```python
from build123d import *

# Parameters (mm, degrees)
SKETCH1_W                      = 40
SKETCH1_H                      = 31
SKETCH1_R                      = 8.75
BOSS_EXTRUDE1_DEPTH            = 19
SHELL1_T                       = -2
SKETCH2_R                      = 10.75
SKETCH2_R_2                    = 8.75
CUT_EXTRUDE1_DEPTH             = 14.5
SKETCH3_W                      = 2
SKETCH3_H                      = 5
BOSS_EXTRUDE2_DEPTH            = 17
SKETCH8_W                      = 7
SKETCH8_H                      = 7
BOSS_EXTRUDE3_DEPTH            = 3
CBORE_FOR_M3_SHCS1_D           = 3.4
CBORE_FOR_M3_SHCS1_CBORE_D     = 6.5
CBORE_FOR_M3_SHCS1_CBORE_DEPTH = 3
CUT_EXTRUDE3_REACH             = 46.125


with BuildPart() as part:
    # Sketch1 → Boss-Extrude1 (new body)
    with BuildSketch(Plane.XY):
        with Locations((-5, 0)):
            Rectangle(SKETCH1_W, SKETCH1_H)
        Circle(SKETCH1_R, mode=Mode.SUBTRACT)
    extrude(amount=-BOSS_EXTRUDE1_DEPTH)

    # Shell1
    shell1_openings = [part.faces().sort_by_distance(p)[0] for p in [
        (-5, -14.993936763, 0),
    ]]
    offset(amount=SHELL1_T, openings=shell1_openings, kind=Kind.INTERSECTION)

    # Sketch2 → Cut-Extrude1 (cut)
    with BuildSketch(Plane.XY):
        with Locations(Location((0, 0, 0), (0, 0, 180))):
            Circle(SKETCH2_R)
        Circle(SKETCH2_R_2, mode=Mode.SUBTRACT)
    extrude(amount=-CUT_EXTRUDE1_DEPTH, mode=Mode.SUBTRACT)

    # Sketch3 → Boss-Extrude2 (add)
    with BuildSketch(Plane.XY.offset(-17)):
        with Locations((-19, 11)):
            Rectangle(SKETCH3_W, SKETCH3_H)
    extrude(amount=BOSS_EXTRUDE2_DEPTH)

    # Sketch8 → Boss-Extrude3 (add)
    with BuildSketch(Plane.XY.offset(-17)):
        with Locations((-14.5, 10)):
            Rectangle(SKETCH8_W, SKETCH8_H)
    extrude(amount=BOSS_EXTRUDE3_DEPTH)

    # CBORE for M3 SHCS1 (through all)
    with Locations(Plane(origin=(0, 0, -19), x_dir=(-1, 0, 0), z_dir=(0, 0, -1))):
        with Locations((15, 10.5)):
            CounterBoreHole(CBORE_FOR_M3_SHCS1_D / 2, CBORE_FOR_M3_SHCS1_CBORE_D / 2, CBORE_FOR_M3_SHCS1_CBORE_DEPTH)

    # Sketch9 → Cut-Extrude3 (cut, up to next)
    with BuildSketch(Plane.XZ.offset(15.5), mode=Mode.PRIVATE) as cut_extrude3_sk1:
        Polygon((-12, 0), (6.5, 0), (9, 0), (9, -3), (6.5, -3), (6.5, -7), (-12, -7), align=None)
    cut_extrude3_tool1 = extrude(cut_extrude3_sk1.sketch, amount=-CUT_EXTRUDE3_REACH, mode=Mode.PRIVATE) & part.part
    add(cut_extrude3_tool1.solids().sort_by_distance((-2.175182, -15.5, -3.390511))[0], mode=Mode.SUBTRACT)


solid = part.part
```
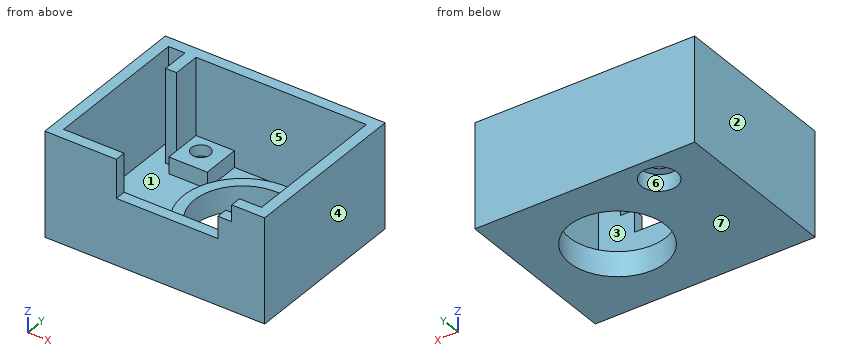
Source: CAD feature listing. Evaluate the final solid. Frame: model axes, mm. Face numbers are marked on the shaded views. A direction names the side the tool comes from. Coordinates: 2 decimals unless noted, no trailing zeros. Loops run counter-clockwise (first coordinate to the right, second up) from the corner with the lowest first, then second, coordinate; pieces in that order, holes last. Notation, with made-up numbers: M 18,80.5 L 62,80.5 A17 ccw 62,104.5 Z; hole C -33.5,84.25 d9. An arc over 180 degrees is marked long. Put each result on its own line as item: value. Start each with the question number.
1) Pull-direction query (X, two-part tool) for the marked faces 1, 2, 3 and 4; classes: pulls with the +X half, pulls with the -X half, needs draft (parallel to the pull), parting line crosses it, or undercut.
2) Cut plane D-D on x = 11.5. Return the cut outline in (y, z), then the cut area to 3 significant figures.
3) Ray query, L1, parallel to Y at x = 0, z = -15.45; L2, parallel to X at y = -13, z = -8.75; L3, parallel to Y at x = 0, z = -18.05. Return the intervals inside material, ascending. Write a range as from..to.
4) Contact query for flat-ended pins moving along their axis: pin 1 Ø5.5 at (x, y) = (-15, 10.5) entering from +Z; pin 2 Ø0.6 at (x, y) = (-7, -14.5) entering from +Z. Output: stop coordinate, or through.
5) Cut plane C-C on z = -4. Return the cut outline in (x, y).
6) Reachability of the marked faces 5, 6 and 7 from +Z, -Z, +X, -X, +Y, -Y: full face, straight path, thin tool, end or side. Return the list, or none.
7) Cut plane A-A on x = 0. Return the cut outline in (y, z).
8) Cut plane B-B on y = 0. Return the cut outline in (x, z).
The answers:
1. face 1: undercut
1. face 2: pulls with the -X half
1. face 3: undercut
1. face 4: pulls with the +X half
2. outline: M -15.5,-19 L 15.5,-19 L 15.5,0 L 13.5,0 L 13.5,-17 L -13.5,-17 L -13.5,0 L -15.5,0 Z
2. area: 130 mm²
3. L1: y = -15.5..-13.5, -10.75..-8.75, 8.75..10.75, 13.5..15.5
3. L2: x = -25..-23, 13..15
3. L3: y = -15.5..-8.75, 8.75..15.5
4. pin 1: stops at z = -14
4. pin 2: stops at z = -7
5. outline: M -25,-15.5 L -12,-15.5 L -12,-13.5 L -23,-13.5 L -23,13.5 L -20,13.5 L -20,8.5 L -18,8.5 L -18,13.5 L 13,13.5 L 13,-13.5 L 6.5,-13.5 L 6.5,-15.5 L 15,-15.5 L 15,15.5 L -25,15.5 Z
6. face 5: +Z
6. face 6: -Z
6. face 7: -Z, +X, -X, +Y, -Y
7. outline: M -15.5,-19 L -8.75,-19 L -8.75,-14.5 L -10.75,-14.5 L -10.75,-17 L -13.5,-17 L -13.5,-7 L -15.5,-7 Z; M 8.75,-19 L 15.5,-19 L 15.5,0 L 13.5,0 L 13.5,-17 L 10.75,-17 L 10.75,-14.5 L 8.75,-14.5 Z
8. outline: M -25,-19 L -8.75,-19 L -8.75,-14.5 L -10.75,-14.5 L -10.75,-17 L -23,-17 L -23,0 L -25,0 Z; M 8.75,-19 L 15,-19 L 15,0 L 13,0 L 13,-17 L 10.75,-17 L 10.75,-14.5 L 8.75,-14.5 Z
